The drawing under review shows one solid part. Ordinate dimensions are in mm from its lowest x, y, z. A direction names the side the tool comes from. Round coordinates to 2 decimals unless told otherwise and drop trailing zeros. Write each loop counter-clockwise with the first axis right and the second up, starting at its lowest first coordinate (ties: lowest second). Pieces come first, ordered by that corner, then holes. Notation, with made-up numbers: (63.25, 86.25) - (80.25, 86.25) arc R7 cw to (80.25, 97.25) - close; hole circle Ø7 at (49.5, -9.5). An arc over 180 degrees is marked (long way). Answer in a Markdown table with one row per item. Add a question column.
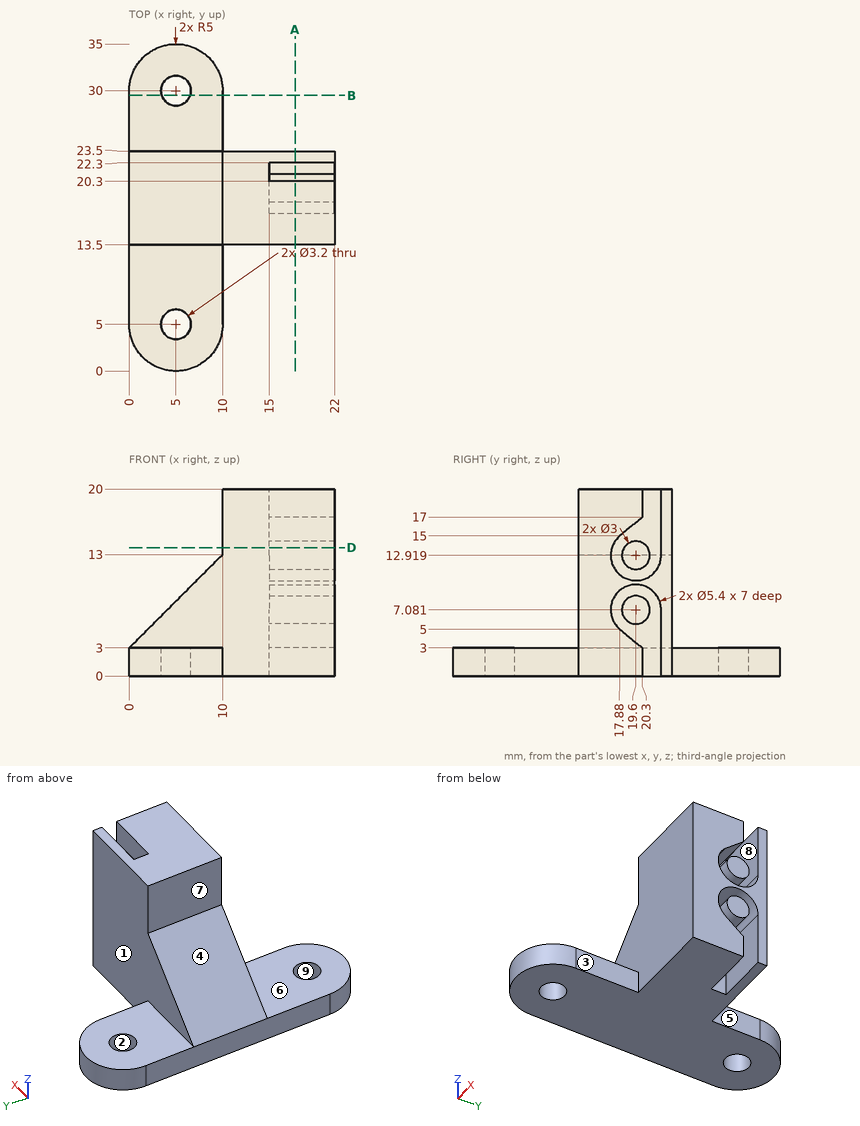
Q1. To check wall thickness, follow probe 1 along Y at (x, z) = (5, 1.55); probe 2 along Z at (x, y) = (17, 20) (1 decimal); probe 3 along X at (y, z) = (30, 1.25). State the ranges of each line that lie inside material, in increasing order.
Q2. Add section D-D on z = 13.75. State the section outline as (x, y) points, then the cut area to 3 significant figures.
Q3. Add section B-B on y = 29.5. State the section outline as (x, z) points.
Q4. Draft analysis for pull direction X (two halves, no side actions). For the marked faces 1, 2, 3 and 4, state which applies: released by +X, released by -X, zero draft, split by the parting line, or undercut.
Q5. Add section A-A on x = 17.75. State the section outline as (y, z) points, then the cut area to 3 significant figures.
Q6. Insertion check: pin 1 Ø5 at (y, z) = (19.6, 12.92) entering from -X; pin 2 Ø3 at (x, y) = (5, 30) entering from +Z; pin 3 Ø2 at (x, z) = (20, 16) entering from -Y; pin 4 Ø4.5 at (y, z) = (19.6, 7.08) entering from -X. Each pin has a flat end and moves straight along its axis. Give the tip position at first contact, or say it passes through.
Q7. Tool access review of the marked faces 5, 6, 7, 8 and 9: name each direction out of +Z, -Z, +X, -X, +Y, -Y from which nothing blocks a thin tool from reaching the whole face with its end or side.
Answer sheet:
| question | item | result |
|---|---|---|
| 1 | probe 1 | y = 0 to 3.4, 6.6 to 28.4, 31.6 to 35 |
| 1 | probe 2 | z = 0 to 3.2, 5.6 to 8.5, 9.8 to 10.2, 11.5 to 14.4, 16.8 to 20 |
| 1 | probe 3 | x = 0 to 3.4, 6.6 to 10 |
| 2 | outline | (10, 13.5) - (22, 13.5) - (22, 17.03) - (15, 17.03) - (15, 18.35) - (22, 18.35) - (22, 20.85) - (15, 20.85) - (15, 22.3) - (22, 22.3) - (22, 23.5) - (10, 23.5) - close |
| 2 | area | 101 mm² |
| 3 | outline | (0, 0) - (3.48, 0) - (3.48, 3) - (0, 3) - close; (6.52, 0) - (10, 0) - (10, 3) - (6.52, 3) - close |
| 4 | face 1 | zero draft |
| 4 | face 2 | undercut |
| 4 | face 3 | released by +X |
| 4 | face 4 | released by -X |
| 5 | outline | (13.5, 0) - (20.3, 0) - (20.3, 3) - (17.88, 5) arc R2.7 cw (long way) to (22.3, 7.08) - (22.3, 0) - (23.5, 0) - (23.5, 20) - (22.3, 20) - (22.3, 12.92) arc R2.7 cw (long way) to (17.88, 15) - (20.3, 17) - (20.3, 20) - (13.5, 20) - close; circle Ø3 at (19.6, 7.08); circle Ø3 at (19.6, 12.92) |
| 5 | area | 145 mm² |
| 6 | pin 1 | stops at x = 7.42 |
| 6 | pin 2 | passes through |
| 6 | pin 3 | stops at y = 13.5 |
| 6 | pin 4 | stops at x = 1.83 |
| 7 | face 5 | +Z, -Z, +X, +Y |
| 7 | face 6 | +Z, +X, -X, -Y |
| 7 | face 7 | +Z, -X, +Y, -Y |
| 7 | face 8 | +Z, +X |
| 7 | face 9 | +Z, -Z |
